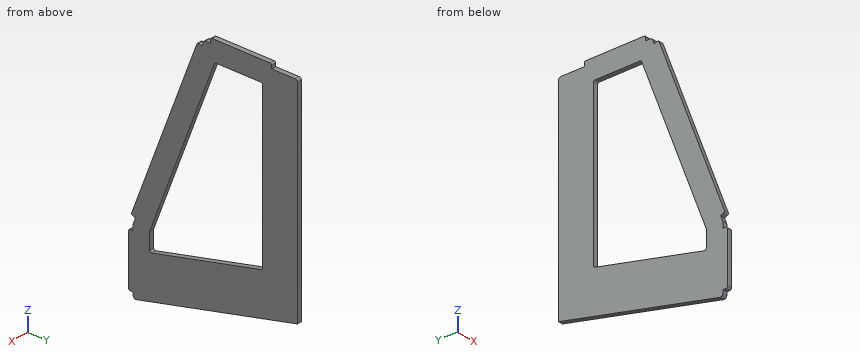
Autodesk Inventor part; units mm, degrees
ref_plane "YZ Plane" through (0, 0, 0) normal (1, 0, 0) x (0, 1, 0)
ref_plane "XZ Plane" through (0, 0, 0) normal (0, 1, 0) x (-1, 0, 0)
ref_plane "XY Plane" through (0, 0, 0) normal (0, 0, 1) x (1, 0, 0)
sketch "Sketch1" plane through (0, 0, 0) normal (1, 0, 0) x (0, 1, 0)
  line L0 (0, 325) -> (0, 0)
  line L1 (0, 0) -> (-211, 0)
  line L2 (-211, 0) -> (-211, 85)
  line L3 (-2.414491, 325) -> (0, 325)
  line L4 (0, 325) -> (-120, 325)
  line L5 (-120, 325) -> (-211, 85)
  dimension "d0" = 325
  dimension "d1" = 211
  dimension "d2" = 85
  dimension "d3" = 120
  dimension "d33" = 240
  dimension "d34" = 91
extrude "Extrusion1" add sketch "Sketch1" along normal blind 6
sketch "Sketch2" plane through (6, 0, 0) normal (1, 0, 0) x (0, 0, -1)
  line L0 (-325, 0) -> (-325, -120)
  line L1 (-325, -33.1) -> (-331, -33.1)
  line L2 (-331, -33.1) -> (-331, -111.9)
  line L3 (-331, -111.9) -> (-325, -111.9)
  line L4 (-325, -111.9) -> (-325, -33.1)
  line L5 (-85, -211) -> (0, -211)
  line L6 (0, -211) -> (0, 0)
  line L7 (-76.9, -211) -> (-8.1, -211)
  line L8 (-8.1, -211) -> (-8.1, -217)
  line L9 (-8.1, -217) -> (-76.9, -217)
  line L10 (-76.9, -217) -> (-76.9, -211)
  line L11 (-325, -120) -> (-331, -111.9) construction
  line L12 (0, 0) -> (-325, 0)
  line L13 (-325, -25) -> (-331, -33.1) construction
  dimension "d6" = 6
  dimension "d12" = 6
  dimension "d13" = 8.1
  dimension "d38" = 25
  dimension "d47" = 8.1
  dimension "d48" = 8.1
extrude "Extrusion2" add sketch "Sketch2" against normal blind 6
sketch "Sketch3" plane through (6, 0, 0) normal (1, 0, 0) x (0, 0, -1)
  line L0 (-317.426159, -122.871748) -> (-92.573841, -208.128252)
  line L1 (-92.573841, -208.128252) -> (-94.701061, -213.738504)
  line L2 (-94.701061, -213.738504) -> (-319.55338, -128.482)
  line L3 (-319.55338, -128.482) -> (-317.426159, -122.871748)
  line L4 (-325, -120) -> (-85, -211)
  dimension "d17" = 8.1
  dimension "d35" = 6
  dimension "d36" = 8.1
extrude "Extrusion3" add sketch "Sketch3" against normal blind 6
sketch "Sketch6" plane through (6, 0, 0) normal (1, 0, 0) x (0, 0, -1)
  line L0 (0, 0) -> (-325, 0)
  line L1 (0, -211) -> (0, 0)
  line L2 (0, -211) -> (-50, 0)
  line L3 (-50, 0) -> (0, 0)
  line L4 (0, -211) -> (0, 0)
  dimension "d39" = 50
extrude "Extrusion6" cut sketch "Sketch6" against normal through all
fillet "Fillet2" radius 3 4 edges at (3, 0, 325) (3, -120, 325) (3, -211, 85) (3, -211, 0)
fillet "Fillet3" radius 2 6 edges at (3, -217, 8.1) (3, -217, 76.9) (3, -213.7385, 94.7011) (3, -128.482, 319.5534) (3, -111.9, 331) (3, -33.1, 331)
sketch "Sketch4" plane through (6, 0, 0) normal (1, 0, 0) x (0, 0, -1)
  line L0 (-323.06361, -120.734214) -> (-85.513953, -210.805126)
  line L1 (-323.06361, -120.734214) -> (-85.513953, -210.805126)
  line L2 (-50, 0) -> (-322, 0)
  line L3 (-325, -3) -> (-325, -33.1)
  line L4 (-325, -33.1) -> (-329, -33.1)
  line L5 (-305, -45) -> (-305, -106.193921)
  line L6 (-305, -106.193921) -> (-84.450343, -189.819)
  line L7 (-84.450343, -189.819) -> (-84.450343, -45)
  line L8 (-84.450343, -45) -> (-305, -45)
  arc A0 (-85.513953, -210.805126) -> (-84.450343, -211) centre (-84.450343, -208) ccw
  point P0 (-191.521346, -165.651434)
  point P1 (-106.085382, -201.605735)
  point P2 (-3, 0)
  point P3 (0, 0)
  dimension "d24" = 45
  dimension "d26" = 20
  dimension "d27" = 20
extrude "Extrusion4" cut sketch "Sketch4" against normal through all
sketch "Sketch7" plane through (6, 0, 0) normal (1, 0, 0) x (0, 0, -1)
  line L0 (-0.874821, -207.308256) -> (-50, 0)
  line L1 (-325, -33.1) -> (-329, -33.1)
  line L2 (-84.450343, -45) -> (-50.133044, -189.819)
  line L3 (-50.133044, -189.819) -> (-84.450343, -189.819)
  line L4 (-84.450343, -45) -> (-84.450343, -189.819)
  point P0 (0, 0)
extrude "Extrusion7" cut sketch "Sketch7" against normal through all
sketch "Sketch8" plane through (6, 0, 0) normal (1, 0, 0) x (0, 0, -1)
  line L0 (-84.450343, -45) -> (-50.133044, -189.819)
  line L1 (-305, -45) -> (-84.450343, -45)
  line L2 (-50.133044, -189.819) -> (-84.450343, -45)
  line L3 (-84.450343, -45) -> (-94.450343, -45)
  line L4 (-94.450343, -45) -> (-60.133044, -189.819)
  line L5 (-50.133044, -189.819) -> (-60.133044, -189.819)
  line L6 (-50.133044, -189.819) -> (-84.450343, -189.819)
  point P0 (0, 0)
  dimension "d44" = 10
extrude "Extrusion8" add sketch "Sketch8" against normal blind 6
fillet "Fillet4" radius 2 5 edges at (3, -189.819, 60.133) (3, -189.819, 84.4503) (3, -45, 94.4503) (3, -106.1939, 305) (3, -45, 305)
equation "\"d26\" = d27"
properties part number "TopSidePanel"
Could you check a few things on this model? Use its own coordinates, in mm. Round coordinates to 2 decimals unless told otherwise and drop trailing zeros. Loops run counter-clockwise (first coordinate to the right, second up) from the corner with the lowest first, then second, coordinate; pieces in that order, holes last. Notation, with made-up numbers: (53.5, -37) -> (58.5, -37) arc R20 ccw to (58.5, -17) -> close; hole circle Ø11 at (29.25, 72.5). An arc over 180 degrees is marked (long way). One line per question, with ' | ' between items.
(1) If we section it at C-C on z = 28: List the corners of the cut face in (x, y) for me.
Model answer:
outline: (0, -217) -> (6, -217) -> (6, -92.84) -> (0, -92.84) -> close
(2) If we section it at B-B on z = 105: List the corners of the cut face in (x, y) for me, and give its area (3 significant figures).
Model answer:
outline: (0, -209.83) -> (6, -209.83) -> (6, -182.03) -> (0, -182.03) -> close; (0, -45) -> (6, -45) -> (6, 0) -> (0, 0) -> close | area: 437 mm^2
(3) If we section it at A-A on y = -78: List the corners of the cut face in (x, z) for me, and give its area (3 significant figures).
Model answer:
outline: (0, 31.52) -> (6, 31.52) -> (6, 86.63) -> (0, 86.63) -> close; (0, 305) -> (6, 305) -> (6, 331) -> (0, 331) -> close | area: 487 mm^2
(4) If I drill on probe 1 along Z at (x, y) = (1.7, -62.5); probe 2 along Z at (x, y) = (3.35, -77); probe 3 along Y at (x, z) = (5.2, 119.5), over which ranges is the centre line in solid material (lowest first)?
Model answer:
probe 1: z = 35.19 to 90.3, 305 to 331 | probe 2: z = 31.75 to 86.87, 305 to 331 | probe 3: y = -204.34 to -176.53, -45 to 0
(5) If we section it at D-D on y = -203: List the corners of the cut face in (x, z) for me.
Model answer:
outline: (0, 1.9) -> (6, 1.9) -> (6, 123.02) -> (0, 123.02) -> close
(6) For pin 1 Ø1 at (x, z) = (3, 296) entering from -Y; pin 2 Ø1.2 at (x, y) = (2.5, -212.5) entering from -Z; pin 3 Ø1.8 at (x, z) = (3, 80) entering from -Y, each with a flat end and sliding along its axis, tell me the tip position at first contact or that it passes through.
Model answer:
pin 1: stops at y = -137.6 | pin 2: stops at z = 8.1 | pin 3: stops at y = -211
